The drawing under review shows one solid part. Ordinate dimensions are in mm from its lowest x, y, z. A direction names the side the tool comes from. Give positions to 0.01 mm unless a question says otherwise; leave off trailing zeros. Write each loop counter-clockwise with the first axis right and the second up, starting at its lowest first coordinate (ties: lowest second). Pieces come first, ordered by that corner, then holes. Notation, with made-up numbers: (-3, 56.5) -> (9, 56.5) arc R20 cw to (9, 70.5) -> close; hole circle Ø4 at (69.5, -5.75). An arc over 180 degrees is marked (long way). Answer as a JSON object with one key per item and string values.
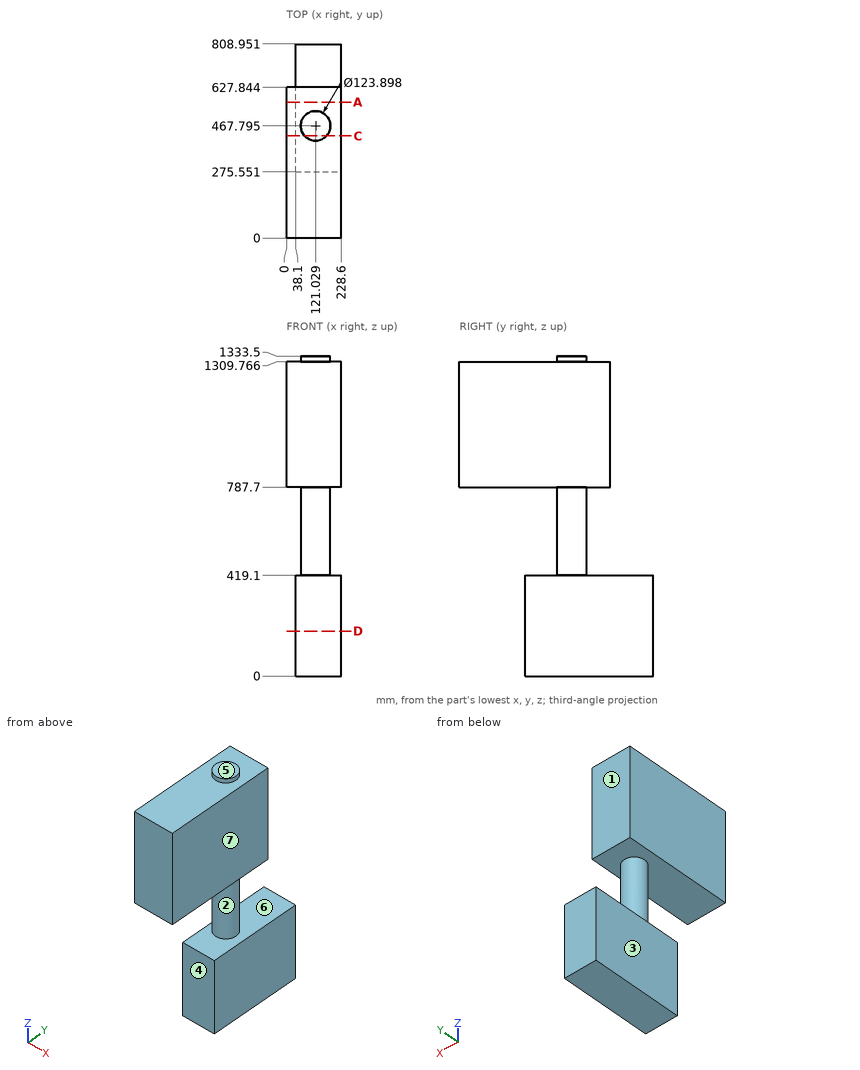
(1) We need section D-D, the plane z = 187.5. State the section outline as (x, y) points.
Here are the results:
{"outline": "(38.1, 275.55) -> (228.6, 275.55) -> (228.6, 808.95) -> (38.1, 808.95) -> close"}
(2) Clearance check with flat-ended pins moving along their axes: pin 1 (4 mm diameter, centred on y = 342, z = 409, fed in from -X); pin 2 (5 mm diameter, centred on x = 29, y = 419.5, fed in from +Z). State where each tip first meets the part, or that it passes through.
Here are the results:
{"pin 1": "stops at x = 38.1", "pin 2": "stops at z = 1309.77"}
(3) For the marked faces 1, 2, 3 and 4, list the 3-axis set-ups (+Z, -Z, +X, -X, +Y, -Y) from which the entire face can be reached by the end or side of a thin tool; tool diameter is ignored.
Here are the results:
{"face 1": "+Z, +X, -X, +Y", "face 2": "none", "face 3": "-Z, -X, +Y, -Y", "face 4": "-Z, +X, -X, -Y"}
(4) We need section A-A, the plane y = 567. State the section outline as (x, z) points (1 decimal).
Here are the results:
{"outline": "(0, 787.7) -> (228.6, 787.7) -> (228.6, 1309.8) -> (0, 1309.8) -> close; (38.1, 0) -> (228.6, 0) -> (228.6, 419.1) -> (38.1, 419.1) -> close"}
(5) For line 1 along Z through (x, y) = (157, 303.5) (1 decimal); line 2 along Z through (x, y) = (59, 649); line 3 along Y through (x, z) = (169, 112.5), list the stretches that pass through material, from the lowest coordinate up.
Here are the results:
{"line 1": "z = 0 to 419.1, 787.7 to 1309.8", "line 2": "z = 0 to 419.1", "line 3": "y = 275.55 to 808.95"}
(6) We need section C-C, the plane y = 425.5. State the section outline as (x, z) points (1 decimal), then the cut area to 3 significant figures.
Here are the results:
{"outline": "(0, 787.7) -> (75.8, 787.7) -> (75.8, 419.1) -> (38.1, 419.1) -> (38.1, 0) -> (228.6, 0) -> (228.6, 419.1) -> (166.3, 419.1) -> (166.3, 787.7) -> (228.6, 787.7) -> (228.6, 1309.8) -> (166.3, 1309.8) -> (166.3, 1333.5) -> (75.8, 1333.5) -> (75.8, 1309.8) -> (0, 1309.8) -> close", "area": "235,000 mm²"}
(7) The part is to be moulded in two halves that separate along Z. For the marked faces 5, 6 and 7, say which applies: +Z half, -Z half, draft (parallel to the pull), parting line (faces both ways), or undercut.
Here are the results:
{"face 5": "+Z half", "face 6": "undercut", "face 7": "draft"}
